from build123d import *

# Parameters (mm, degrees)
SKETCH1_W                                = 83
SKETCH1_H                                = 83
BOSS_EXTRUDE1_DEPTH                      = 6
SKETCH2_R                                = 1.5
CUT_EXTRUDE1_DEPTH                       = 118.532974097
SKETCH5_W                                = 50.5
SKETCH5_H                                = 34
BOSS_EXTRUDE2_DEPTH                      = 22
SKETCH6_W                                = 44.5
SKETCH6_H                                = 28
CUT_EXTRUDE5_DEPTH                       = 25
FILLET1_R                                = 3
SKETCH8_R                                = 12.5
CUT_EXTRUDE6_DEPTH                       = 10
CUT_EXTRUDE7_DEPTH                       = 121.673112167
CUT_EXTRUDE7_DEPTH_BACK                  = 121.673112167
SKETCH9_W                                = 83
SKETCH9_H                                = 8
CUT_EXTRUDE8_DEPTH                       = 3
MIRROR1_AT_THE_SECOND_PLANE_COPY_1_DEPTH = 3
CUT_EXTRUDE9_DEPTH                       = 14
CUT_EXTRUDE10_DEPTH                      = 10
CUT_EXTRUDE11_DEPTH                      = 10
BOSS_EXTRUDE3_DEPTH                      = 3
CUT_EXTRUDE14_DEPTH                      = 4
SKETCH20_W                               = 13.564659966
SKETCH20_H                               = 7
CUT_EXTRUDE15_DEPTH                      = 4
BOSS_EXTRUDE4_DEPTH                      = 4
BOSS_EXTRUDE4_DEPTH_BACK                 = 1
SKETCH21_W                               = 27.5
SKETCH21_H                               = 37
FILLET2_R                                = 5


with BuildPart() as part:
    # Sketch1 → Boss-Extrude1 (new body)
    with BuildSketch(Plane(origin=(0, 0, 0), x_dir=(1, 0, 0), z_dir=(0, 1, 0))):
        with Locations((41.5, 41.5)):
            Rectangle(SKETCH1_W, SKETCH1_H)
    extrude(amount=BOSS_EXTRUDE1_DEPTH)

    # Sketch2 → Cut-Extrude1 (cut, through all)
    with BuildSketch(Plane(origin=(0, 6, 0), x_dir=(1, 0, 0), z_dir=(0, 1, 0))):
        with Locations(Location((6, 71, 0), (0, 0, 270))):
            Circle(SKETCH2_R)
        with Locations(Location((6, 12, 0), (0, 0, 270))):
            Circle(SKETCH2_R)
        with Locations(Location((77, 12, 0), (0, 0, 270))):
            Circle(SKETCH2_R)
        with Locations(Location((77, 71, 0), (0, 0, 270))):
            Circle(SKETCH2_R)
    extrude(amount=-CUT_EXTRUDE1_DEPTH, mode=Mode.SUBTRACT)

    # Sketch5 → Boss-Extrude2 (add)
    with BuildSketch(Plane(origin=(0, 6, 0), x_dir=(1, 0, 0), z_dir=(0, 1, 0))):
        with Locations((34, 17)):
            Rectangle(SKETCH5_W, SKETCH5_H)
    extrude(amount=BOSS_EXTRUDE2_DEPTH)

    # Sketch6 → Cut-Extrude5 (cut)
    with BuildSketch(Plane(origin=(0, 28, 0), x_dir=(1, 0, 0), z_dir=(0, 1, 0))):
        with Locations((34, 17)):
            Rectangle(SKETCH6_W, SKETCH6_H)
    extrude(amount=-CUT_EXTRUDE5_DEPTH, mode=Mode.SUBTRACT)

    # Fillet1
    fillet1_edges = [part.edges().sort_by_distance(p)[0] for p in [
        (59.25, 17, -34),
        (8.75, 17, -34),
        (8.75, 17, 0),
        (59.25, 17, 0),
    ]]
    fillet(fillet1_edges, radius=FILLET1_R)

    # Sketch8 → Cut-Extrude6 (cut)
    with BuildSketch(Plane.XY):
        with Locations((41.5, 13.5)):
            Circle(SKETCH8_R)
    extrude(amount=-CUT_EXTRUDE6_DEPTH, mode=Mode.SUBTRACT)

    # Sketch9 → Cut-Extrude7 (cut, two sides: drawn at the far end of the back side and taken through both)
    with BuildSketch(Plane.XY.offset(-CUT_EXTRUDE7_DEPTH_BACK)):
        with Locations((41.5, 24)):
            Rectangle(SKETCH9_W, SKETCH9_H)
    extrude(amount=CUT_EXTRUDE7_DEPTH + CUT_EXTRUDE7_DEPTH_BACK, mode=Mode.SUBTRACT)

    # Sketch11 → Cut-Extrude8 (cut)
    with BuildSketch(Plane.XZ):
        Polygon((3, -9), (13, -9), (13, -15), (8, -21), (3, -21), align=None)
    cut_extrude8 = extrude(amount=-CUT_EXTRUDE8_DEPTH, mode=Mode.SUBTRACT)

    # Mirror1: Cut-Extrude8 across plane
    add(cut_extrude8.mirror(Plane.XY.offset(-41.5)), mode=Mode.SUBTRACT)

    # Mirror1 at the second plane: Cut-Extrude8 across plane
    add(cut_extrude8.mirror(Plane.ZY.offset(-41.5)), mode=Mode.SUBTRACT)

    # Mirror1 at the second plane copy 1 sketc → Mirror1 at the second plane copy 1 (cut)
    with BuildSketch(Plane(origin=(83, 0, -83), x_dir=(-1, 0, 0), z_dir=(0, -1, 0))):
        Polygon((3, -9), (13, -9), (13, -15), (8, -21), (3, -21), align=None)
    extrude(amount=-MIRROR1_AT_THE_SECOND_PLANE_COPY_1_DEPTH, mode=Mode.SUBTRACT)

    # Sketch13 → Cut-Extrude9 (cut)
    with BuildSketch(Plane(origin=(0, 20, 0), x_dir=(1, 0, 0), z_dir=(0, 1, 0))):
        with BuildLine():
            Line((11.75, 8.007820144), (11.75, 15.992179856))
            ThreePointArc((11.75, 15.992179856), (10.422332723, 17.426137972), (8.75, 18.437196595))
            Line((8.75, 18.437196595), (8.75, 5.562803405))
            ThreePointArc((8.75, 5.562803405), (10.422332723, 6.573862028), (11.75, 8.007820144))
        make_face()
    extrude(amount=-CUT_EXTRUDE9_DEPTH, mode=Mode.SUBTRACT)

    # Sketch14 → Cut-Extrude10 (cut)
    with BuildSketch(Plane.XY):
        Polygon((29, 13.5), (29, 20), (30.822921748, 20), align=None)
    extrude(amount=-CUT_EXTRUDE10_DEPTH, mode=Mode.SUBTRACT)

    # Sketch15 → Cut-Extrude11 (cut)
    with BuildSketch(Plane.XY):
        Polygon((54, 20), (54, 13.5), (52.177078252, 20), align=None)
    extrude(amount=-CUT_EXTRUDE11_DEPTH, mode=Mode.SUBTRACT)

    # Sketch17 → Boss-Extrude3 (add)
    with BuildSketch(Plane.XZ):
        Polygon((9.666666667, -9), (9.666666667, -19), (13, -15), (13, -9), align=None)
    extrude(amount=-BOSS_EXTRUDE3_DEPTH)

    # Sketch18 → Cut-Extrude14 (cut)
    with BuildSketch(Plane(origin=(0, 3, 0), x_dir=(1, 0, 0), z_dir=(0, 1, 0))):
        Polygon((34.717670017, 3), (34.717670017, 10), (48.282329983, 10), (48.282329983, 3), (56.25, 3), (56.25, 31), (11.75, 31), (11.75, 3), align=None)
    extrude(amount=-CUT_EXTRUDE14_DEPTH, mode=Mode.SUBTRACT)

    # Sketch20 → Cut-Extrude15 (cut)
    with BuildSketch(Plane.XZ):
        with Locations((41.5, -6.5)):
            Rectangle(SKETCH20_W, SKETCH20_H)
    extrude(amount=-CUT_EXTRUDE15_DEPTH, mode=Mode.SUBTRACT)

    # Sketch21 → Boss-Extrude4 (add, two sides: drawn at the far end of the back side and taken through both)
    with BuildSketch(Plane.XZ.offset(-BOSS_EXTRUDE4_DEPTH_BACK)):
        with Locations((47.5, -18.5)):
            Rectangle(SKETCH21_W, SKETCH21_H)
    extrude(amount=BOSS_EXTRUDE4_DEPTH + BOSS_EXTRUDE4_DEPTH_BACK)

    # Fillet2
    fillet2_edges = [part.edges().sort_by_distance(p)[0] for p in [
        (33.75, -2, -37),
        (61.25, -2, -37),
    ]]
    fillet(fillet2_edges, radius=FILLET2_R)


solid = part.part
For this review, take the finished solid that the model builds, in its own axes (mm). A direction names the side the tool comes from. Coordinates: 2 decimals unless noted, no trailing zeros. Order: outer loops, then holes, each group sorted by start corner. A loop starts at its lowest first (then second) coordinate and runs counter-clockwise, first axis right, second up. Notation, with made-up numbers: (-22, 48) -> (31, 48) arc R14 ccw to (31, 72) -> close; hole circle Ø2 at (-16, 26). An arc over 180 degrees is marked (long way). Return JSON: item names as keys, results as strings.
1. We need section C-C on x = 77. Write out the cut boundary in (y, z), and give its area (3 significant figures).
Answer block:
{"outline": "(0, -83) -> (6, -83) -> (6, -72.5) -> (3, -72.5) -> (3, -74) -> (0, -74) -> close; (0, -62) -> (3, -62) -> (3, -69.5) -> (6, -69.5) -> (6, -13.5) -> (3, -13.5) -> (3, -21) -> (0, -21) -> close; (0, -9) -> (3, -9) -> (3, -10.5) -> (6, -10.5) -> (6, 0) -> (0, 0) -> close", "area": "408 mm²"}
2. For pin 1 Ø2 at (x, y) = (21.5, 15) entering from -Z; pin 2 Ø11 at (x, z) = (6, -67.5) entering from -Y; pin 3 Ø4 at (x, z) = (67, -60.5) entering from +Y; pin 4 Ø8 at (y, z) = (10.5, -72) entering from +X, all flat-tipped, find the tip position at first contact; note any pin that passes through.
Answer block:
{"pin 1": "z = -34", "pin 2": "y = 0", "pin 3": "y = 6", "pin 4": "through"}
3. We need section D-D on z = -12. State how many separate pieces and enclosed holes the cut face has, and give its area (4 significant figures).
Answer block:
{"separate pieces": "4", "enclosed holes": "0", "area": "337.5 mm²"}
4. We need section A-A on z = -71. Write out the cut boundary in (x, y).
Answer block:
{"outline": "(0, 0) -> (3, 0) -> (3, 3) -> (4.5, 3) -> (4.5, 6) -> (0, 6) -> close; (7.5, 3) -> (13, 3) -> (13, 0) -> (70, 0) -> (70, 3) -> (75.5, 3) -> (75.5, 6) -> (7.5, 6) -> close; (78.5, 3) -> (80, 3) -> (80, 0) -> (83, 0) -> (83, 6) -> (78.5, 6) -> close"}
5. The part is to be moulded in two halves that separate along X. For faces 1 (the cylindrical face through (9.61, 13.1, -33.1)), 2 (the cylindrical face through (58.39, 13.1, -33.1)), 3 (the cylindrical face through (41.225, 1.003, -1.479)), 4 (the flat face through (6, 1, -62)), say which applies: +X half, -X half, draft (parallel to the pull), parting line (faces both ways), or undercut.
Answer block:
{"face 1": "-X half", "face 2": "+X half", "face 3": "undercut", "face 4": "undercut"}
6. For line 1 (X direction, y = 3.85, z = -12); line 2 (X direction, y = 0.75, z = -72.5); line 3 (X direction, y = 2.75, z = -12.5), list the stretches that pass through material, from the lowest coordinate up. Write a range as from..to.
Answer block:
{"line 1": "0..4.5, 7.5..11.75, 56.25..75.5, 78.5..83", "line 2": "0..3, 13..70, 80..83", "line 3": "0..3, 9.67..11.75, 56.25..70, 80..83"}
7. Machinability: for faces 5 (the flat face through (29, 17, -1)), 6 (the cylindrical face through (58.35, 13.1, -0.86)), 7 (the flat face through (59.25, 13, -17)), 8 (the cylindrical face through (59.75, -2.03, -35.57)), which of the approach directions +Z, -Z, +X, -X, +Y, -Y give a long, thin tool a straight path to every point of the face, cutting with its end or side? Answer none if there is none.
Answer block:
{"face 5": "+Z, +Y", "face 6": "+Z, +X, +Y", "face 7": "+Z, -Z, +X, +Y", "face 8": "-Z, +X, -Y"}
8. We need section B-B on y = 15. Write out the cut boundary in (x, z), and give its area (3 significant figures).
Answer block:
{"outline": "(8.75, -31) arc R3 ccw to (11.75, -34) -> (56.25, -34) arc R3 ccw to (59.25, -31) -> (59.25, -3) arc R3 ccw to (56.25, 0) -> (54, 0) -> (54, -3) -> (56.25, -3) -> (56.25, -31) -> (11.75, -31) -> (11.75, -15.99) arc R7 cw to (8.75, -18.44) -> close; (8.75, -5.56) arc R7 cw to (11.75, -8.01) -> (11.75, -3) -> (29, -3) -> (29, 0) -> (11.75, 0) arc R3 ccw to (8.75, -3) -> close", "area": "356 mm²"}
